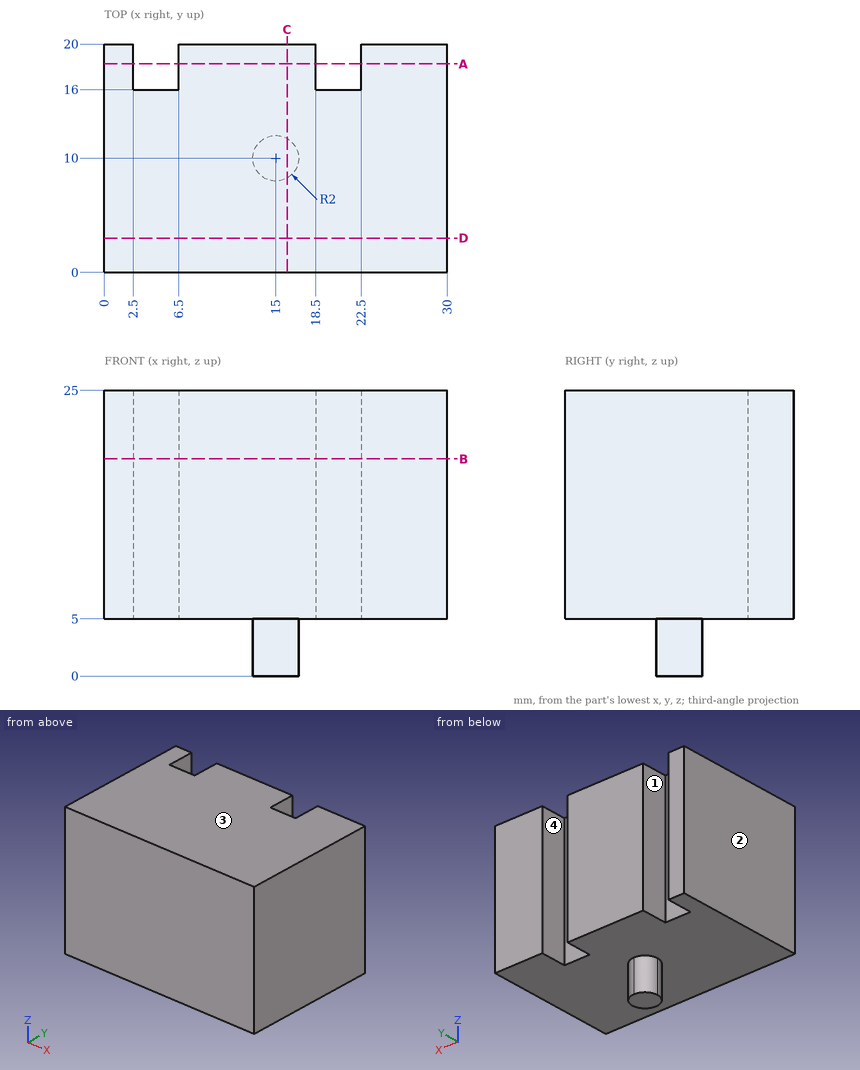
Study the drawing (mm; zero at the part's minimum x, y, z) and answer. Give positions to 0.01 mm unless a question says otherwise; leave off trailing zeros. Loops run counter-clockwise (first coordinate to the right, second up) from the corner with the lowest first, then second, coordinate; pieces in that order, holes last. Notation, with made-up numbers: (-35.75, 34.25) - (-23.75, 34.25) arc R26 ccw to (-23.75, 62.25) - close; hole circle Ø6 at (31, -2.75). An arc over 180 degrees is marked (long way). Answer as CSV lines item,"result". Start each with the question number.
1) Find section A-A (y = 18.25). Write down the section's boundary in (x, z).
2) Find section D-D (y = 3). Write down the section's boundary in (x, z), then the cut area to 3 significant figures.
3) Determine the mould class of the marked faces 1, 2, 3 and 4 for opening direction X: released by +X, released by -X, zero draft, split by the parting line, or undercut.
4) Straight lines are drawn through the part: L1, parallel to X at y = 16.75, z = 9; L2, parallel to Z at x = 7.75, y = 12.25; L3, parallel to Y at x = 5.5, z = 5.5. For each, find the intervals that lie inside material, in ascending order. Write a range as from..to.
5) Find section B-B (z = 19). Write down the section's boundary in (x, y), then the cut area to 3 significant figures.
6) Each of these flat-tipped pins is pushed along its axis until it touches: pin 1 Ø10 at (y, z) = (3.5, 21.5) entering from -X; pin 2 Ø2 at (x, z) = (4, 18.5) entering from +Y; pin 3 Ø5 at (x, y) = (25.5, 5) entering from -Z. Where does it stop, or does it pass through?
7) Find section C-C (x = 16). Write down the section's boundary in (y, z), then the cut area to 3 significant figures.
Findings below:
1,outline,"(0, 5) - (2.5, 5) - (2.5, 25) - (0, 25) - close; (6.5, 5) - (18.5, 5) - (18.5, 25) - (6.5, 25) - close; (22.5, 5) - (30, 5) - (30, 25) - (22.5, 25) - close"
2,outline,"(0, 5) - (30, 5) - (30, 25) - (0, 25) - close"
2,area,"600 mm^2"
3,face 1,"undercut"
3,face 2,"released by -X"
3,face 3,"zero draft"
3,face 4,"undercut"
4,L1,"0..2.5, 6.5..18.5, 22.5..30"
4,L2,"5..25"
4,L3,"0..16"
5,outline,"(0, 0) - (30, 0) - (30, 20) - (22.5, 20) - (22.5, 16) - (18.5, 16) - (18.5, 20) - (6.5, 20) - (6.5, 16) - (2.5, 16) - (2.5, 20) - (0, 20) - close"
5,area,"568 mm^2"
6,pin 1,"x = 0"
6,pin 2,"y = 16"
6,pin 3,"z = 5"
7,outline,"(0, 5) - (8.27, 5) - (8.27, 0) - (11.73, 0) - (11.73, 5) - (20, 5) - (20, 25) - (0, 25) - close"
7,area,"417 mm^2"
